```python
from build123d import *

# Parameters (mm, degrees)
ESQUISSE1_R             = 4
BOSS_EXTRU_1_DEPTH      = 65
ESQUISSE2_R             = 1.5
ENL_V_MAT_EXTRU_1_DEPTH = 5
CONG_1_R                = 1


with BuildPart() as part:
    # Esquisse1 → Boss.-Extru.1 (new body)
    with BuildSketch(Plane.XY):
        Circle(ESQUISSE1_R)
    extrude(amount=BOSS_EXTRU_1_DEPTH)

    # Esquisse2 → Enlèv. mat.-Extru.1 (cut, symmetric)
    with BuildSketch(Plane(origin=(0, 0, 0), x_dir=(0, 0, -1), z_dir=(1, 0, 0))):
        with Locations(Location((-25.5, 0, 0), (0, 0, 179.999999999))):
            Circle(ESQUISSE2_R)
        with Locations(Location((-4.5, 0, 0), (0, 0, 179.999999999))):
            Circle(ESQUISSE2_R)
    extrude(amount=ENL_V_MAT_EXTRU_1_DEPTH, both=True, mode=Mode.SUBTRACT)

    # Congé1
    cong_1_edges = [part.edges().sort_by_distance(p)[0] for p in [
        (-4, 0, 65),
    ]]
    fillet(cong_1_edges, radius=CONG_1_R)


solid = part.part
```
Input: part model. Units: mm. Frame: model coordinates. Coordinates: 2 decimals unless noted, no trailing zeros. Write each loop counter-clockwise with the first axis right and the second up, starting at its lowest first coordinate (ties: lowest second). Pieces come first, ordered by that corner, then holes. Notation, with made-up numbers: (-10.75, 81.25) - (-6.75, 81.25) arc R28 cw to (-6.75, 105.25) - close; hole circle Ø7 at (-1.75, 54.25). An arc over 180 degrees is marked (long way). Put each result on its own line as item: value. Start each with the question number.
1) Cut plane C-C (x = -2). State how many separate pieces and enclosed holes the cut face has, plus the area to 3 significant figures.
2) Cut plane B-B (z = 4.5). Return the cut outline in (x, y), plus the area to 3 significant figures.
3) Contact query for flat-ended pins moving along their axis: pin 1 (1 mm diameter, centred on x = -1, y = 1.5, fed in from -Z); pin 2 (3 mm diameter, centred on y = -3, z = 26.5, fed in from -X). Output: stop coordinate, or through.
4) Cut plane D-D (z = 29). Return the cut outline in (x, y).
5) Ray query, L1, parallel to Z at x = 2.5, y = -1; L2, parallel to Y at x = 3.05, z = 25.5; L3, parallel to Y at x = 1.25, z = 4.5. Return the intervals inside material, ascending.
6) Mould query, pull axis X, two halves, no side actions, for faces 1 (the face through (3.695, -1.532, 31.552)), 2 (the face through (0, 0, 65)). Classes: pulls with the +X half, pulls with the -X half, needs draft (parallel to the pull), parting line crosses it, or undercut.
7) Cut plane A-A (y = 0). Return the cut outline in (x, z), plus the area to 3 significant figures.
Resolved:
1. separate pieces: 1
1. enclosed holes: 2
1. area: 436 mm2
2. outline: (-3.71, -1.5) arc R4 ccw to (3.71, -1.5) - close; (-3.71, 1.5) - (3.71, 1.5) arc R4 ccw to start
2. area: 26.8 mm2
3. pin 1: stops at z = 0
3. pin 2: stops at x = -3.71
4. outline: circle Ø8 at (0, 0)
5. L1: z = 0 to 3.38, 5.62 to 24.38, 26.62 to 65
5. L2: y = -2.59 to -1.5, 1.5 to 2.59
5. L3: y = -3.8 to -1.5, 1.5 to 3.8
6. face 1: parting line crosses it
6. face 2: needs draft
7. outline: (-4, 0) - (4, 0) - (4, 3) - (-4, 3) - close; (-4, 6) - (4, 6) - (4, 24) - (-4, 24) - close; (-4, 27) - (4, 27) - (4, 64) arc R1 ccw to (3, 65) - (-3, 65) arc R1 ccw to (-4, 64) - close
7. area: 472 mm2
